Could you check a few things on this model? Use its own coordinates, in mm. Round coordinates to 2 decimals unless told otherwise and drop trailing zeros. Order: outer loops, then holes, each group sorted by start corner. A loop starts at its lowest first (then second) coordinate and runs counter-clockwise, first axis right, second up. Notation, with made-up numbers: M 15.5,9 L 45.5,9 A26 cw 45.5,41 Z; hole C 38.5,42.5 d7. An arc over 180 degrees is marked long. Write each question's results on one line, items separated by ' | '. Start each with the question number.
1. I'm going to push flat-ended pins straight in: pin 1 (2.5 mm diameter, centred on x = 721.5, y = 0.5, fed in from +Z); pin 2 (1.5 mm diameter, centred on x = 459, y = 4, fed in from -Z); pin 3 (3 mm diameter, centred on x = 120.5, y = -5, fed in from +Z). Where does each tip first touch, or does it pass through?
2. Suppose I cut it at A-A on x = 381.5. Write out the boundary of the cut face in (y, z), and give its area (3 significant figures).
3. Please list where these lines run through material, in increasing order: L1, parallel to Z at x = 50, y = -7.8; L2, parallel to Y at x = 157.5, z = -1; L3, parallel to X at y = -4, z = -183.
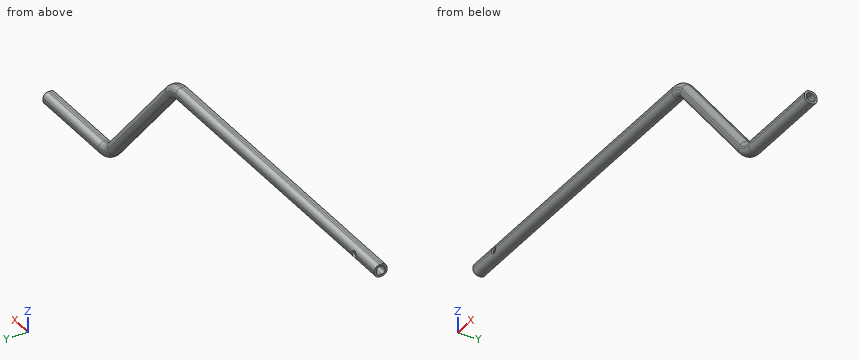
from build123d import *

# Parameters (mm, degrees)
CUT_EXTRUDE3_DEPTH      = 836.299457856
CUT_EXTRUDE3_DEPTH_BACK = 836.299457856
SKETCH21_R              = 5


with BuildPart() as part:
    # Sweep-Thin3: sweep along a curve in space
    with BuildLine() as sweep_thin3_path:
        Line((674.686132166, 0, -191.51111078), (810.696902422, 0, -191.51111078))
        ThreePointArc((651.704798873, 0, -180.79473907), (662.007584314, 0, -188.700344391), (674.686132166, 0, -191.51111078))
        Line((508.992103549, 0, -10.716371709), (651.704798873, 0, -180.79473907))
        ThreePointArc((486.010770255, 0, 0), (498.689318108, 0, -2.810766389), (508.992103549, 0, -10.716371709))
        Line((0, 0, 0), (486.010770255, 0, 0))
    # Sketch2 → Sweep-Thin3 (sweep)
    with BuildSketch(Plane(origin=(0, 0, 0), x_dir=(0, 0, -1), z_dir=(1, 0, 0))):
        with BuildLine():
            Line((1.5, 9.5), (-1.5, 9.5))
            ThreePointArc((-1.5, 9.5), (-7.156854249, 7.156854249), (-9.5, 1.5))
            Line((-9.5, 1.5), (-9.5, -1.5))
            ThreePointArc((-9.5, -1.5), (-7.156854249, -7.156854249), (-1.5, -9.5))
            Line((-1.5, -9.5), (1.5, -9.5))
            ThreePointArc((1.5, -9.5), (7.156854249, -7.156854249), (9.5, -1.5))
            Line((9.5, -1.5), (9.5, 1.5))
            ThreePointArc((9.5, 1.5), (7.156854249, 7.156854249), (1.5, 9.5))
        make_face()
        with BuildLine():
            Line((1.5, 6.5), (-1.5, 6.5))
            ThreePointArc((-1.5, 6.5), (-5.035533906, 5.035533906), (-6.5, 1.5))
            Line((-6.5, 1.5), (-6.5, -1.5))
            ThreePointArc((-6.5, -1.5), (-5.035533906, -5.035533906), (-1.5, -6.5))
            Line((-1.5, -6.5), (1.5, -6.5))
            ThreePointArc((1.5, -6.5), (5.035533906, -5.035533906), (6.5, -1.5))
            Line((6.5, -1.5), (6.5, 1.5))
            ThreePointArc((6.5, 1.5), (5.035533906, 5.035533906), (1.5, 6.5))
        make_face(mode=Mode.SUBTRACT)
    sweep(path=sweep_thin3_path.line)

    # Sketch21 → Cut-Extrude3 (cut, two sides: drawn at the far end of the back side and taken through both)
    with BuildSketch(Plane(origin=(0, 0, 0), x_dir=(1, 0, 0), z_dir=(0, 1, 0)).offset(-CUT_EXTRUDE3_DEPTH_BACK)):
        with Locations(Location((50, 0, 0), (0, 0, 197.457603124))):
            Circle(SKETCH21_R)
    extrude(amount=CUT_EXTRUDE3_DEPTH + CUT_EXTRUDE3_DEPTH_BACK, mode=Mode.SUBTRACT)


solid = part.part
Filled sheet:
1) pin 1: stops at z = -182.01 | pin 2: stops at z = -9.31 | pin 3: stops at z = 9.25
2) outline: M -9.5,-1.5 A8 ccw -1.5,-9.5 L 1.5,-9.5 A8 ccw 9.5,-1.5 L 9.5,1.5 A8 ccw 1.5,9.5 L -1.5,9.5 A8 ccw -9.5,1.5 Z; hole M -6.5,-1.5 A5 ccw -1.5,-6.5 L 1.5,-6.5 A5 ccw 6.5,-1.5 L 6.5,1.5 A5 ccw 1.5,6.5 L -1.5,6.5 A5 ccw -6.5,1.5 Z | area: 159 mm^2
3) L1: z = -6.43 to -5, 5 to 6.43 | L2: y = -9.5 to -6.5, 6.5 to 9.5 | L3: x = 641.68 to 645.94, 663.62 to 810.7
